Read the model definition and answer for the solid it produces. Units are mm, in the model's axes. A direction names the side the tool comes from. Coordinates: 2 decimals unless noted, no trailing zeros. Write each loop counter-clockwise with the first axis right and the second up, starting at its lowest first coordinate (ties: lowest second). Pieces come first, ordered by that corner, then holes. Notation, with made-up numbers: M 51.25,72 L 78.25,72 A19 cw 78.25,107 Z; hole C 84.5,-17 d7. An arc over 180 degrees is marked long. Write item = value, one per line.
from build123d import *

# Parameters (mm, degrees)
RING_DEPTH              = 2.653567955
RING_DEPTH_BACK         = 0.508
SKETCH2_R               = 29.138416471
SKETCH2_R_2             = 20.83618439
TEETH_START             = -0.401310706
SKETCH4_W               = 7.816761814
SKETCH4_H               = 9.871955338
TEETH_DEPTH             = 3.054878706
CIRPATTERN1_COUNT       = 5
SKETCH6_R               = 3.416225964
CUT_EXTRUDE1_DEPTH      = 8.89
CIRPATTERN2_COUNT       = 5
CUT_EXTRUDE3_DEPTH      = 7.874
CUT_EXTRUDE3_DEPTH_BACK = 5.08
SKETCH7_R               = 12.218567197


with BuildPart() as part:
    # Sketch2 → Ring (new, two sides: drawn at the far end of the back side and taken through both)
    with BuildSketch(Plane.XY.offset(-RING_DEPTH_BACK)):
        Circle(SKETCH2_R)
        Circle(SKETCH2_R_2, mode=Mode.SUBTRACT)
    extrude(amount=RING_DEPTH + RING_DEPTH_BACK)

    # Sketch4 → Teeth (add)
    with BuildSketch(Plane.XY.offset(TEETH_START)):
        with Locations((0, 15.900206721)):
            Rectangle(SKETCH4_W, SKETCH4_H)
    teeth = extrude(amount=TEETH_DEPTH)

    # CirPattern1: Teeth ×5 about axis
    cirpattern1_axis = Axis((0, 0, 0), (0, 0, 1))
    for i in range(1, CIRPATTERN1_COUNT):
        add(teeth.rotate(cirpattern1_axis, i * 360 / CIRPATTERN1_COUNT))

    # Sketch6 → Cut-Extrude1 (cut)
    with BuildSketch(Plane(origin=(0, 0, -0.508), x_dir=(-1, 0, 0), z_dir=(0, 0, -1))):
        with Locations((-23.307220113, 7.528711947)):
            Circle(SKETCH6_R)
    cut_extrude1 = extrude(amount=-CUT_EXTRUDE1_DEPTH, mode=Mode.SUBTRACT)

    # CirPattern2: Cut-Extrude1 ×5 about axis
    cirpattern2_axis = Axis((0, 0, 0), (0, 0, 1))
    for i in range(1, CIRPATTERN2_COUNT):
        add(cut_extrude1.rotate(cirpattern2_axis, i * 360 / CIRPATTERN2_COUNT), mode=Mode.SUBTRACT)

    # Sketch7 → Cut-Extrude3 (cut, two sides: drawn at the far end of the back side and taken through both)
    with BuildSketch(Plane.XY.offset(-CUT_EXTRUDE3_DEPTH_BACK)):
        with Locations((0, 0.340402239)):
            Circle(SKETCH7_R)
    extrude(amount=CUT_EXTRUDE3_DEPTH + CUT_EXTRUDE3_DEPTH_BACK, mode=Mode.SUBTRACT)


solid = part.part
Item 1: Find section A-A (x = 8). Determine the outline of the cut face in (y, z).
Worked answers:
outline = M -28.02,-0.51 L -19.24,-0.51 L -19.24,2.65 L -28.02,2.65 Z; M -17.66,-0.4 L -8.9,-0.4 L -8.9,2.65 L -17.66,2.65 Z; M 19.24,-0.51 L 28.02,-0.51 L 28.02,2.65 L 19.24,2.65 Z
Item 2: Flat-ended cylindrical pins translate along their axes: pin 1 (1.5 mm diameter, centred on x = -3, y = 11, fed in from -Z); pin 2 (8.5 mm diameter, centred on x = -1.5, y = 16, fed in from -Z); pin 3 (1 mm diameter, centred on y = 6.5, z = 2, fed in from +X); pin 4 (1.5 mm diameter, centred on y = 21.5, z = 0.5, fed in from -X). Find the tip coordinate at first contact, or state that the pin passes through.
Worked answers:
pin_1 = through
pin_2 = -0.4
pin_3 = 28.51
pin_4 = -20.46
Item 3: Find section C-C (x = -22). Determine the outline of the cut face in (y, z), and give its area (3 significant figures).
Worked answers:
outline = M -19.11,-0.51 L 4.44,-0.51 L 4.44,2.65 L -19.11,2.65 Z; M 10.78,-0.51 L 19.11,-0.51 L 19.11,2.65 L 10.78,2.65 Z
area = 101 mm²
Item 4: Consider line 1 along Y through (x, z) = (13.5, -0.05); line 2 along Y through (x, z) = (-13, 1.55); line 3 along Y through (x, z) = (8.5, 1.35). Determine where each line is inside the solid, lowest interval first. Write a range as from..to.
Worked answers:
line_1 = -25.82..-23.15, -16.53..-11.93, 0.28..8.5, 15.87..25.82
line_2 = -26.08..-22.89, -16.69..-11.24, 0.11..8.33, 16.28..26.08
line_3 = -27.87..-19.02, -18.35..-8.44, 19.02..27.87
Item 5: Find section D-D (z = 0.6). Determine the outline of the cut face in (x, y).
Worked answers:
outline = C 0,0 d58.28; hole C -23.28,7.61 d6.83; hole M -20.67,2.61 A20.84 ccw -15.19,-14.26 L -9.84,-6.9 A12.22 ccw -3.44,-11.38 L -8.87,-18.85 A20.84 ccw 8.87,-18.85 L 3.44,-11.38 A12.22 ccw 9.84,-6.9 L 15.19,-14.26 A20.84 ccw 20.67,2.61 L 12.21,-0.14 A12.22 ccw 10,7.36 L 18.26,10.04 A20.84 ccw 3.91,20.47 L 3.91,11.92 A12.22 ccw -3.91,11.92 L -3.91,20.47 A20.84 ccw -18.26,10.04 L -10,7.36 A12.22 ccw -12.21,-0.14 Z; hole C -14.43,-19.79 d6.83; hole C 0.04,24.49 d6.83; hole C 14.36,-19.84 d6.83; hole C 23.31,7.53 d6.83
Item 6: Find section B-B (y = 1). Determine the outline of the cut face in (x, z).
Worked answers:
outline = M -29.12,-0.51 L -20.81,-0.51 L -20.81,2.65 L -29.12,2.65 Z; M -15.73,-0.4 L -12.2,-0.4 L -12.2,2.65 L -15.73,2.65 Z; M 12.2,-0.4 L 15.73,-0.4 L 15.73,2.65 L 12.2,2.65 Z; M 20.81,-0.51 L 29.12,-0.51 L 29.12,2.65 L 20.81,2.65 Z
Item 7: Which of the six approach directions +Z, -Z, +X, -X, +Y, -Y give full straight-line access (tool end or side, diameter ignored) to faces 4 (the face through (16.381, 1.213, 1.105)), 5 (the face through (-15, 5, -0.401)), 6 (the face through (19, 9, -0.508))?
Worked answers:
face_4 = +Z, -Z
face_5 = -Z
face_6 = -Z, +X, -X, +Y, -Y
Item 8: For a pull along Y with two mould halves and no side action, classify faces 1 (the face through (0, 16, -0.401)), 2 (the face through (4.3, -11.8, 2.654)), 3 (the face through (-11.706, 3.843, 1.105)) as released by +Y, released by -Y, zero draft, split by the parting line, or undercut.
Worked answers:
face_1 = undercut
face_2 = zero draft
face_3 = undercut
